Could you check a few things on this model? Use its own coordinates, in mm. Face numbers are marked on the shaded views. A direction names the side the tool comes from. Round coordinates to 2 decimals unless told otherwise and drop trailing zeros. Loops run counter-clockwise (first coordinate to the right, second up) from the corner with the lowest first, then second, coordinate; pieces in that order, holes last. Notation, with made-up numbers: (87.5, 82.5) - (93.5, 82.5) arc R19 ccw to (93.5, 103.5) - close; hole circle Ø1 at (37, 29). An arc over 180 degrees is marked (long way). Use one line per item in the form item = value.
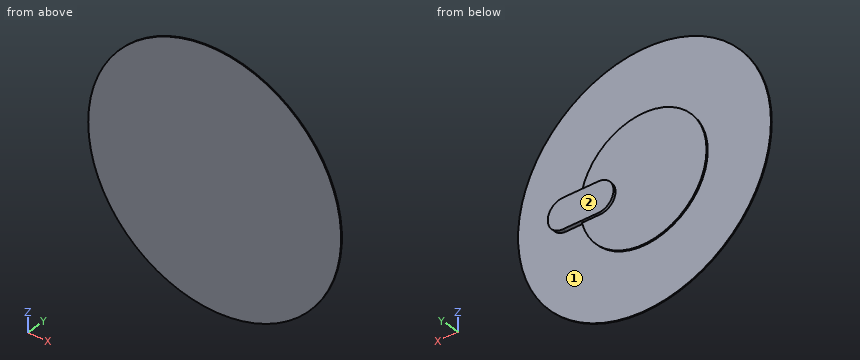
```python
from build123d import *

# Parameters (mm, degrees)
SKETCH_R             = 25
PAD_DEPTH            = 0.2
SKETCH001_R          = 12.5
PAD001_DEPTH         = 0.5
PAD002_DEPTH         = 1
BODY_PLACEMENT_ANGLE = 180


with BuildPart() as part:
    # Sketch → Pad (new body)
    with BuildSketch(Plane.XZ):
        Circle(SKETCH_R)
    extrude(amount=PAD_DEPTH)

    # Sketch001 → Pad001 (join)
    with BuildSketch(Plane.XZ):
        Circle(SKETCH001_R)
    extrude(amount=PAD001_DEPTH)

    # Sketch002 → Pad002 (join)
    with BuildSketch(Plane.XZ):
        with BuildLine():
            ThreePointArc((-15.5, 3), (-18.5, 0), (-15.5, -3))
            Line((-15.5, -3), (-8.5, -3))
            ThreePointArc((-8.5, -3), (-5.5, 0), (-8.5, 3))
            Line((-15.5, 3), (-8.5, 3))
        make_face()
    extrude(amount=PAD002_DEPTH)


with BuildPart() as part_1:
    # Body placement: moved
    add(part.part.moved(Location((0, 1, 0))).rotate(Axis((0, 1, 0), (0, 0, 1)), BODY_PLACEMENT_ANGLE))


solid = part_1.part
```
1. If we section it at C-C, the plane y = 1.8: Write out the boundary of the cut face in (x, z).
Solution:
outline = (8.5, -3) - (15.5, -3) arc R3 ccw to (15.5, 3) - (8.5, 3) arc R3 ccw to start
2. Please list where these lines run through material, in increasing order: line 1 along Y through (x, z) = (7, 3.5); line 2 along Y through (x, z) = (-6.5, -15.5); line 3 along Z through (x, y) = (10, 1.8).
Solution:
line_1 = 1 to 1.5
line_2 = 1 to 1.2
line_3 = -3 to 3
3. On a 3-axis mill with a long thin cutter (end or side, diameter ignored), from which of +Z, -Z, +X, -X, +Y, -Y can I reach the whole of each face in a straight line? I mean the marked faces 1 and 2. Say none if no direction works.
Solution:
face_1 = +Y
face_2 = +Z, -Z, +X, -X, +Y
4. If we section it at D-D, the plane x = 6.5: Write out the boundary of the cut face in (y, z).
Solution:
outline = (1, -24.14) - (1.2, -24.14) - (1.2, -10.68) - (1.5, -10.68) - (1.5, -2.24) - (2, -2.24) - (2, 2.24) - (1.5, 2.24) - (1.5, 10.68) - (1.2, 10.68) - (1.2, 24.14) - (1, 24.14) - close
5. For P1, Ø19.5, axis at x = -4.5, z = 0, coming from the +Y side, with a flat end and sliding along its axis, tell me the tip position at first contact or that it passes through.
Solution:
P1 = 1.5
6. If we section it at A-A, the plane z = 0: Write out the boundary of the cut face in (x, y), plus the area to 3 significant figures.
Solution:
outline = (-25, 1) - (25, 1) - (25, 1.2) - (18.5, 1.2) - (18.5, 2) - (5.5, 2) - (5.5, 1.5) - (-12.5, 1.5) - (-12.5, 1.2) - (-25, 1.2) - close
area = 25.8 mm^2
7. If we section it at B-B, the plane x = 0: Write out the boundary of the cut face in (y, z).
Solution:
outline = (1, -25) - (1.2, -25) - (1.2, -12.5) - (1.5, -12.5) - (1.5, 12.5) - (1.2, 12.5) - (1.2, 25) - (1, 25) - close
